Work out the finished part from the listing and answer in its coordinate system (mm). A direction names the side the tool comes from. Round coordinates to 2 decimals unless told otherwise and drop trailing zeros. Write each loop counter-clockwise with the first axis right and the second up, starting at its lowest first coordinate (ties: lowest second). Pieces come first, ordered by that corner, then holes. Notation, with made-up numbers: M -25,-8.5 L -14,-8.5 A20 cw -14,17.5 Z; hole C 64.25,-5 d5. An arc over 180 degrees is marked long. Answer in a Markdown table with one row per item.
```python
from build123d import *

# Parameters (mm, degrees)
EXTRUDE1_REACH = 8.88


with BuildPart() as part:
    # Sketch1 → base-Revolve (revolve)
    with BuildSketch(Plane.XY, mode=Mode.PRIVATE) as base_revolve_sk:
        Polygon((0, 1.9558), (-0.254, 1.9558), (-0.254, 1.524), (-1.524, 1.524), (-1.524, 1.2192), (-1.27, 1.2192), (-1.27, 0), (0, 0), (4.7752, 0), (4.7752, 0.762), (0, 0.762), align=None)
    revolve(base_revolve_sk.sketch.rotate(Axis((0, 0, 0), (1, 0, 0)), 90), axis=Axis((0, 0, 0), (1, 0, 0)))

    # Sketch15 → Extrude1 (add, up to next)
    with BuildSketch(Plane.ZY.offset(1.524), mode=Mode.PRIVATE) as extrude1_sk1:
        with BuildLine():
            ThreePointArc((-1.319822717, -0.761999997), (-1.524, 6e-09), (-1.319822711, 0.762000008))
            Line((-1.319822711, 0.762000008), (-1.75976362, 0))
            Line((-1.75976362, 0), (-1.319822717, -0.761999997))
        make_face()
    extrude1_tool1 = extrude(extrude1_sk1.sketch, amount=-EXTRUDE1_REACH, mode=Mode.PRIVATE) - part.part
    # Sketch15 → Extrude1 (add, up to next)
    with BuildSketch(Plane.ZY.offset(1.524), mode=Mode.PRIVATE) as extrude1_sk2:
        with BuildLine():
            ThreePointArc((-1.319822711, 0.762000008), (-0.761999998, 1.319822717), (-5e-09, 1.524))
            Line((-5e-09, 1.524), (-0.87988181, 1.524))
            Line((-0.87988181, 1.524), (-1.319822711, 0.762000008))
        make_face()
    extrude1_tool2 = extrude(extrude1_sk2.sketch, amount=-EXTRUDE1_REACH, mode=Mode.PRIVATE) - part.part
    # Sketch15 → Extrude1 (add, up to next)
    with BuildSketch(Plane.ZY.offset(1.524), mode=Mode.PRIVATE) as extrude1_sk3:
        with BuildLine():
            ThreePointArc((-5e-09, 1.524), (0.761999979, 1.319822727), (1.319822694, 0.762000038))
            Line((1.319822694, 0.762000038), (0.87988181, 1.524))
            Line((0.87988181, 1.524), (-5e-09, 1.524))
        make_face()
    extrude1_tool3 = extrude(extrude1_sk3.sketch, amount=-EXTRUDE1_REACH, mode=Mode.PRIVATE) - part.part
    # Sketch15 → Extrude1 (add, up to next)
    with BuildSketch(Plane.ZY.offset(1.524), mode=Mode.PRIVATE) as extrude1_sk4:
        with BuildLine():
            Line((1.319822721, -0.76199999), (1.75976362, 0))
            Line((1.75976362, 0), (1.319822694, 0.762000038))
            ThreePointArc((1.319822694, 0.762000038), (1.472070954, 0.394440246), (1.524, 0))
            ThreePointArc((1.524, 0), (1.472070961, -0.394440219), (1.319822721, -0.76199999))
        make_face()
    extrude1_tool4 = extrude(extrude1_sk4.sketch, amount=-EXTRUDE1_REACH, mode=Mode.PRIVATE) - part.part
    # Sketch15 → Extrude1 (add, up to next)
    with BuildSketch(Plane.ZY.offset(1.524), mode=Mode.PRIVATE) as extrude1_sk5:
        with BuildLine():
            Line((0.87988181, -1.524), (1.319822721, -0.76199999))
            ThreePointArc((1.319822721, -0.76199999), (0.762000003, -1.319822714), (-5e-09, -1.524))
            Line((-5e-09, -1.524), (0.87988181, -1.524))
        make_face()
    extrude1_tool5 = extrude(extrude1_sk5.sketch, amount=-EXTRUDE1_REACH, mode=Mode.PRIVATE) - part.part
    # Sketch15 → Extrude1 (add, up to next)
    with BuildSketch(Plane.ZY.offset(1.524), mode=Mode.PRIVATE) as extrude1_sk6:
        with BuildLine():
            Line((-0.87988181, -1.524), (-5e-09, -1.524))
            ThreePointArc((-5e-09, -1.524), (-0.762000004, -1.319822713), (-1.319822717, -0.761999997))
            Line((-1.319822717, -0.761999997), (-0.87988181, -1.524))
        make_face()
    extrude1_tool6 = extrude(extrude1_sk6.sketch, amount=-EXTRUDE1_REACH, mode=Mode.PRIVATE) - part.part
    add(extrude1_tool1.solids().sort_by_distance((-1.524, 0, -1.57515))[0])
    add(extrude1_tool2.solids().sort_by_distance((-1.524, 1.36412, -0.787575))[0])
    add(extrude1_tool3.solids().sort_by_distance((-1.524, 1.36412, 0.787575))[0])
    add(extrude1_tool4.solids().sort_by_distance((-1.524, 0, 1.57515))[0])
    add(extrude1_tool5.solids().sort_by_distance((-1.524, -1.36412, 0.787575))[0])
    add(extrude1_tool6.solids().sort_by_distance((-1.524, -1.36412, -0.787575))[0])

    # Sketch8 → point_Cut-Revolve1 (revolve, cut)
    with BuildSketch(Plane.XY, mode=Mode.PRIVATE) as point_cut_revolve1_sk:
        Polygon((4.7752, 0), (5.2832, 0), (5.2832, 1.27), (4.137285688, 1.27), (4.137285688, 0.762), (4.7752, 0.3937), align=None)
    revolve(point_cut_revolve1_sk.sketch.rotate(Axis((0, 0, 0), (1, 0, 0)), 90), axis=Axis((0, 0, 0), (1, 0, 0)), mode=Mode.SUBTRACT)


solid = part.part
```
1. The part is cut by section B-B (x = -1). Determine the outline of the cut face in (y, z).
Calculated:
| item | result |
|---|---|
| outline | M -1.52,-0.88 L 0,-1.76 L 1.52,-0.88 L 1.52,0.88 L 0,1.76 L -1.52,0.88 Z |
2. The part is cut by section A-A (z = 0). Determine the outline of the cut face in (x, y), plus the area to 3 significant figures.
Calculated:
| item | result |
|---|---|
| outline | M -1.52,-1.52 L -0.25,-1.52 L -0.25,-1.96 L 0,-1.96 L 0,-0.76 L 4.14,-0.76 L 4.78,-0.39 L 4.78,0.39 L 4.14,0.76 L 0,0.76 L 0,1.96 L -0.25,1.96 L -0.25,1.52 L -1.52,1.52 L -1.52,1.22 L -1.27,1.22 L -1.27,-1.22 L -1.52,-1.22 Z |
| area | 11.3 mm² |
3. A tool of negligible diameter and unlimited length cuts with its end or side. For faces 4 (the flat face through (0, 1, 0)), 5 (the flat face through (-1.524, -1, 1)), 6 (the flat face through (-1, -1.524, 0)), from which of +Z, -Z, +X, -X, +Y, -Y can it reach the whole face along a straight path? Write none if from no direction.
Calculated:
| item | result |
|---|---|
| face 4 | +X |
| face 5 | +Z, -Z, -X, +Y, -Y |
| face 6 | +Z, -Z, -X, -Y |
4. Consider line 1 along Y through (x, z) = (-1.35, 0); line 2 along X through (y, z) = (-1.1, 0.25); line 3 along X through (y, z) = (-0.2, 0.1). Determine where each line is inside the solid, lowest interval first. Write a range as from..to.
Calculated:
| item | result |
|---|---|
| line 1 | y = -1.52..-1.22, 1.22..1.52 |
| line 2 | x = -1.27..0 |
| line 3 | x = -1.27..4.78 |
5. Given pin 1 (1.4 mm diameter, centred on x = -1, z = -0.5, fed in from +Y); pin 2 (0.6 mm diameter, centred on x = -1, z = 0, fed in from -Y), each flat-ended and moving along its own axis, determine where each tip first touches the part or whether it passes through.
Calculated:
| item | result |
|---|---|
| pin 1 | stops at y = 1.52 |
| pin 2 | stops at y = -1.52 |
6. The part is cut by section D-D (z = 1.4). Determine the outline of the cut face in (x, y), plus the area to 3 significant figures.
Calculated:
| item | result |
|---|---|
| outline | M -1.52,-0.62 L -0.25,-0.62 L -0.25,-1.37 L 0,-1.37 L 0,1.37 L -0.25,1.37 L -0.25,0.62 L -1.52,0.62 Z |
| area | 2.28 mm² |
7. Determine the mould class of faces 1 (the flat face through (-1, 1.524, 0)), 2 (the flat face through (-1.27, 0, 0)), 3 (the cylindrical face through (2.04, -0.756, -0.099)) for opening direction Z: released by +Z, released by -Z, zero draft, split by the parting line, or undercut.
Calculated:
| item | result |
|---|---|
| face 1 | zero draft |
| face 2 | undercut |
| face 3 | split by the parting line |
8. The part is cut by section C-C (y = 1.35). Determine the outline of the cut face in (x, z).
Calculated:
| item | result |
|---|---|
| outline | M -1.52,-0.98 L -0.25,-0.98 L -0.25,-1.42 L 0,-1.42 L 0,1.42 L -0.25,1.42 L -0.25,0.98 L -1.52,0.98 Z |
